Verification items for the finished model (mm, model axes). Give positions to 0.01 mm unless a question says otherwise; leave off trailing zeros. Write each loop counter-clockwise with the first axis right and the second up, starting at its lowest first coordinate (ties: lowest second). Pieces come first, ordered by that corner, then holes. Notation, with made-up numbers: (-18, 56.25) -> (29, 56.25) arc R27 ccw to (29, 94.25) -> close; hole circle Ø7 at (12.25, -38). An arc over 180 degrees is marked (long way). Use one line per item in the form item = value. Start each with the question number.
(1) Section check A-A, the plane x = 0. Record the cut outline in (y, z) (3 decimals), plus the area to 3 significant figures.
(2) Scan lines: L1, parallel to Z at x = -0.15, y = -0.4; L2, parallel to X at y = 0.05, z = 4.5; L3, parallel to X at y = 0, z = 10.5 (3 decimals). Record each from-to range of solid material in increasing order.
(3) Section check C-C, the plane z = 6.5. Record the cut outline in (x, y) (3 decimals), plus the area to 3 significant figures.
(4) Section check B-B, the plane z = 2. Record the cut outline in (x, y), plus the area to 3 significant figures.
from build123d import *

# Parameters (mm, degrees)
SKETCH1_R               = 0.5
BOSS_EXTRUDE1_DEPTH     = 5
SKETCH1_3_R             = 0.375
BOSS_EXTRUDE2_DEPTH     = 11
CHAMFER1_SIZE           = 0.062
CUT_EXTRUDE1_DEPTH      = 12.022703843
CUT_EXTRUDE1_DEPTH_BACK = 12.022703843
SKETCH2_W               = 0.74
SKETCH2_H               = 0.05859


with BuildPart() as part:
    # Sketch1 → Boss-Extrude1 (new body)
    with BuildSketch(Plane.XY):
        Circle(SKETCH1_R)
    extrude(amount=BOSS_EXTRUDE1_DEPTH)

    # Sketch1<3> → Boss-Extrude2 (add)
    with BuildSketch(Plane.XY):
        Circle(SKETCH1_3_R)
    extrude(amount=BOSS_EXTRUDE2_DEPTH)

    # Chamfer1
    chamfer1_edges = [part.edges().sort_by_distance(p)[0] for p in [
        (-0.375, 0, 11),
    ]]
    chamfer(chamfer1_edges, length=CHAMFER1_SIZE)

    # Sketch2 → Cut-Extrude1 (cut, two sides: drawn at the far end of the back side and taken through both)
    with BuildSketch(Plane(origin=(0, 0, 0), x_dir=(0, 0, -1), z_dir=(1, 0, 0)).offset(-CUT_EXTRUDE1_DEPTH_BACK)):
        Rectangle(SKETCH2_W, SKETCH2_H)
    extrude(amount=CUT_EXTRUDE1_DEPTH + CUT_EXTRUDE1_DEPTH_BACK, mode=Mode.SUBTRACT)


solid = part.part
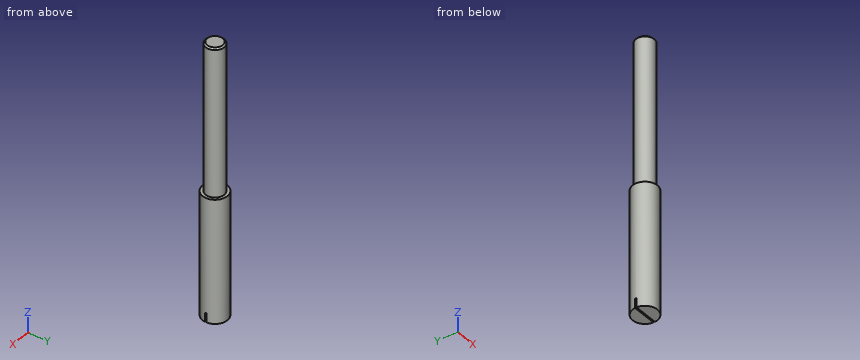
Completed:
q1.outline = (-0.5, 0) -> (-0.029, 0) -> (-0.029, 0.37) -> (0.029, 0.37) -> (0.029, 0) -> (0.5, 0) -> (0.5, 5) -> (0.375, 5) -> (0.375, 10.938) -> (0.313, 11) -> (-0.313, 11) -> (-0.375, 10.938) -> (-0.375, 5) -> (-0.5, 5) -> close
q1.area = 9.47 mm²
q2.L1 = 0 to 5
q2.L2 = -0.5 to 0.5
q2.L3 = -0.375 to 0.375
q3.outline = circle Ø0.75 at (0, 0)
q3.area = 0.442 mm²
q4.outline = circle Ø1 at (0, 0)
q4.area = 0.785 mm²
